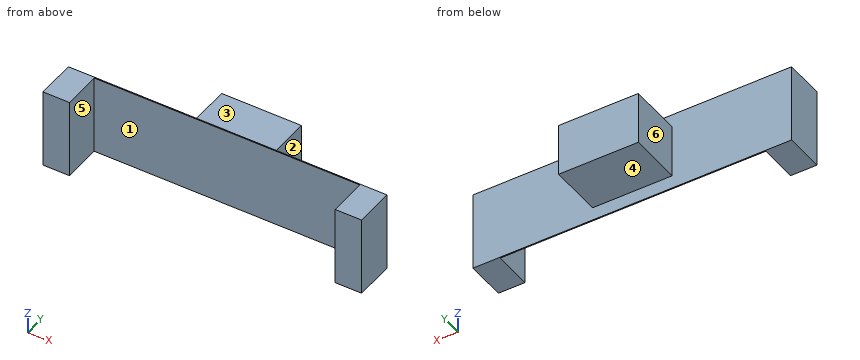
Autodesk Inventor part; units mm, degrees
ref_plane "YZ Plane" through (0, 0, 0) normal (1, 0, 0) x (0, 1, 0)
ref_plane "XZ Plane" through (0, 0, 0) normal (0, 1, 0) x (-1, 0, 0)
ref_plane "XY Plane" through (0, 0, 0) normal (0, 0, 1) x (1, 0, 0)
sketch "Sketch1" plane through (0, 0, 0) normal (0, 0, 1) x (1, 0, 0)
  line L0 (0, 0) -> (5, 0)
  line L1 (5, 0) -> (5, 7.3)
  line L2 (5, 7.5) -> (0, 7.5)
  line L3 (0, 7.5) -> (0, 0)
  line L4 (5, 7.5) -> (55, 7.5)
  line L5 (55, 7.5) -> (55, 7.3)
  line L6 (55, 7.3) -> (5, 7.3)
  line L7 (5, 7.3) -> (5, 7.5)
  line L8 (55, 7.5) -> (60, 7.5)
  line L9 (60, 7.5) -> (60, 0)
  line L10 (60, 0) -> (55, 0)
  line L11 (55, 0) -> (55, 7.5)
  dimension "d0" = 5
  dimension "d1" = 7.5
  dimension "d2" = 50
  dimension "d3" = 0.2
  dimension "d4" = 5
  dimension "d5" = 7.5
extrude "Extrusion1" add sketch "Sketch1" along normal blind 15
sketch "Sketch2" plane through (0, 7.5, 0) normal (0, 1, 0) x (1, 0, 0)
  line L0 (0, 0) -> (0, -15)
  line L1 (0, -7.5) -> (30, -7.5) construction
  line L2 (60, 0) -> (60, -15)
  line L3 (30, -7.5) -> (30, 0) construction
  line L4 (5, 0) -> (55, 0)
  line L5 (22.5, -12.5) -> (37.5, -12.5)
  line L6 (37.5, -12.5) -> (37.5, -2.5)
  line L7 (37.5, -2.5) -> (22.5, -2.5)
  line L8 (22.5, -2.5) -> (22.5, -12.5)
  line L9 (22.5, -12.5) -> (37.5, -2.5) construction
  line L10 (37.5, -12.5) -> (22.5, -2.5) construction
  dimension "d8" = 30
  dimension "d9" = 15
  dimension "d10" = 10
extrude "Extrusion2" add sketch "Sketch2" along normal blind 10
properties part number "bridgeTest"
Check sheet for the modelled part. Datum: model origin and axes. Units: mm. Face numbers are marked on the shaded views. A direction names the side the tool comes from. Give positions to 0.01 mm unless a question says otherwise; leave off trailing zeros. Loops run counter-clockwise (first coordinate to the right, second up) from the corner with the lowest first, then second, coordinate; pieces in that order, holes last. Notation, with made-up numbers: M -24.75,32.5 L 14.25,32.5 A17 ccw 14.25,54.5 Z; hole C 41.5,-2.5 d4. An arc over 180 degrees is marked long. Use a Markdown table: item, result. Add a question column.
Q1. Sectioned sample at C-C, the plane x = 26. Record the cut outline in (y, z), then the cut area to 3 significant figures.
Q2. Sectioned sample at A-A, the plane y = 5.25. Record the cut outline in (x, z), then the cut area to 3 significant figures.
Q3. Go/stop test with flat-tipped pins: pin 1 (4 mm diameter, centred on x = 32, y = 15, fed in from -Z); pin 2 (5 mm diameter, centred on y = 13, z = 7, fed in from -X); pin 3 (1.5 mm diameter, centred on x = 21.5, z = 9.5, fed in from -Y). Record where each tip stops, or that it passes through.
Q4. Sectioned sample at D-D, the plane z = 1.75. Record the cut outline in (x, y), then the cut area to 3 significant figures.
Q5. Sectioned sample at B-B, the plane z = 4.75. Record the cut outline in (x, y), then the cut area to 3 significant figures.
Q6. Scan lines: line 1 along X through (y, z) = (6.5, 0.5); line 2 along Y through (x, z) = (22, 7.25); line 3 along Z through (x, y) = (36, 8.5). Record each from-to range of solid material in increasing order. Write a range as [from, to].
Q7. Tool access check on the marked faces 4, 5 and 6. Record the directions out of +Z, -Z, +X, -X, +Y, -Y that give a thin tool (end or side, any length) a straight path to the whole face; none if there is none.
Q8. Mould release check, pull along X, two halves, no side actions. Record for the marked faces 1, 2 and 3: pulls with the +X half, pulls with the -X half, needs draft (parallel to the pull), parting line crosses it, or undercut.
Verdict:
| question | item | result |
|---|---|---|
| 1 | outline | M 7.3,0 L 7.5,0 L 7.5,2.5 L 17.5,2.5 L 17.5,12.5 L 7.5,12.5 L 7.5,15 L 7.3,15 Z |
| 1 | area | 103 mm^2 |
| 2 | outline | M 0,0 L 5,0 L 5,15 L 0,15 Z; M 55,0 L 60,0 L 60,15 L 55,15 Z |
| 2 | area | 150 mm^2 |
| 3 | pin 1 | z = 2.5 |
| 3 | pin 2 | x = 22.5 |
| 3 | pin 3 | y = 7.3 |
| 4 | outline | M 0,0 L 5,0 L 5,7.3 L 55,7.3 L 55,0 L 60,0 L 60,7.5 L 0,7.5 Z |
| 4 | area | 85.0 mm^2 |
| 5 | outline | M 0,0 L 5,0 L 5,7.3 L 55,7.3 L 55,0 L 60,0 L 60,7.5 L 37.5,7.5 L 37.5,17.5 L 22.5,17.5 L 22.5,7.5 L 0,7.5 Z |
| 5 | area | 235 mm^2 |
| 6 | line 1 | [0, 5], [55, 60] |
| 6 | line 2 | [7.3, 7.5] |
| 6 | line 3 | [2.5, 12.5] |
| 7 | face 4 | -Z, +X, -X, +Y |
| 7 | face 5 | +Z, -Z, -Y |
| 7 | face 6 | +Z, -Z, -X, +Y |
| 8 | face 1 | undercut |
| 8 | face 2 | pulls with the +X half |
| 8 | face 3 | needs draft |
